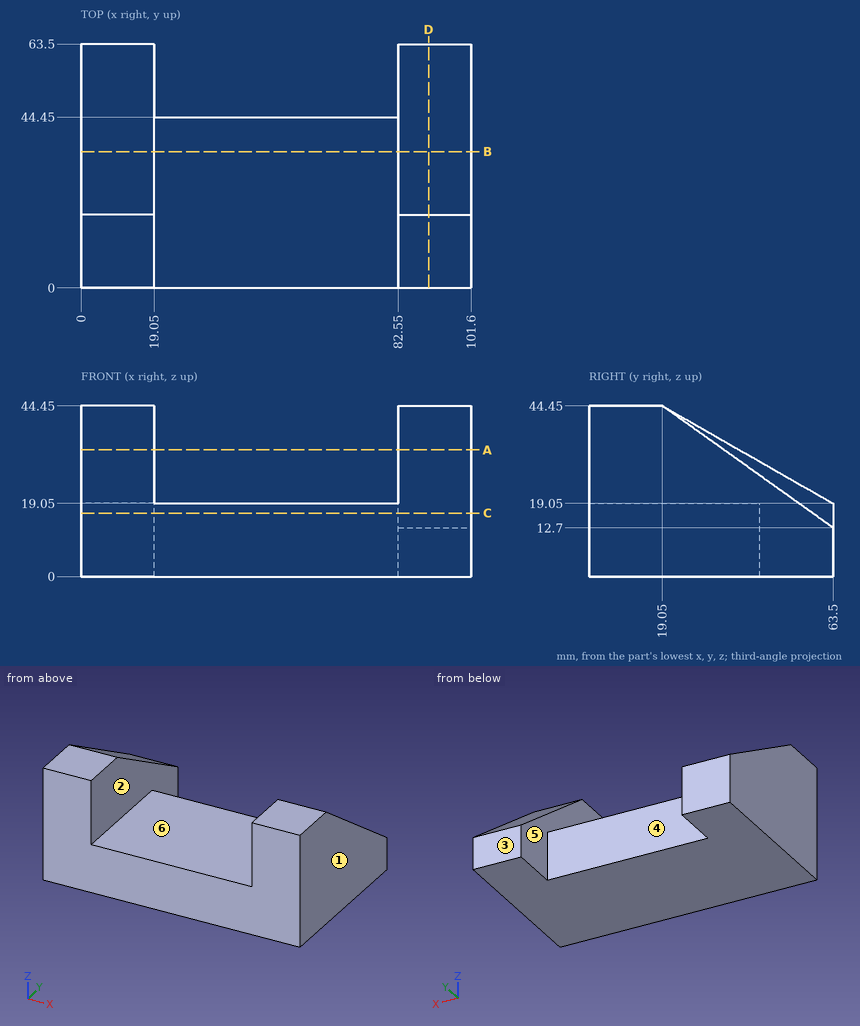
Design review of the part shown in the three views and the two pictorial views. Dimensions are in mm from the part's minimum x, y and z. A direction names the side the tool comes from. Give positions to 0.01 mm unless a question says otherwise; leave off trailing zeros. Loops run counter-clockwise (first coordinate to the right, second up) from the corner with the lowest first, then second, coordinate; pieces in that order, holes last. Notation, with made-up numbers: M 21.5,-18.5 L 71.5,-18.5 A20 cw 71.5,10.5 Z; hole C -36,-23 d3. An arc over 180 degrees is marked long. Answer as a JSON object with one key per item and string values. Group by question number.
Q1. For probe 1 along X at (y, z) = (16, 20.5); probe 2 along Y at (x, z) = (35.5, 10); probe 3 along Z at (x, y) = (81.5, 34), list the stretches that pass through material, from the lowest coordinate up. Write a range as [from, to].
Q2. Add section C-C on z = 16.5. Give the boundary of the cut face in (x, y), and give its area (3 significant figures).
Q3. Mouldability with a two-part tool opening along X and no side actions: class the marked faces 1, 2 and 3 as +X half, -X half, draft (parallel to the pull), parting line (faces both ways), or undercut.
Q4. Add section B-B on y = 35.5. Give the boundary of the cut face in (x, z).
Q5. Add section A-A on z = 33. Give the boundary of the cut face in (x, y), and give its area (3 significant figures).
Q6. Insertion check: P1, Ø5.5, axis at x = 43.5, z = 11, coming from the +Y side. The pin has a flat end and moves straight along its axis. Give the tip position at first contact, or say it passes through.
Q7. Add section D-D on x = 90.5. Give the boundary of the cut face in (y, z).
Q8. Tool access review of the marked faces 4, 5 and 6: name each direction out of +Z, -Z, +X, -X, +Y, -Y from which nothing blocks a thin tool from reaching the whole face with its end or side.
Checked values:
{
 "1": {"probe 1": "[0, 19.05], [82.55, 101.6]", "probe 2": "[0, 44.45]", "probe 3": "[0, 19.05]"},
 "2": {"outline": "M 0,0 L 101.6,0 L 101.6,58.18 L 82.55,58.18 L 82.55,44.45 L 19.05,44.45 L 19.05,63.5 L 0,63.5 Z", "area": "5,140 mm²"},
 "3": {"face 1": "+X half", "face 2": "undercut", "face 3": "draft"},
 "4": {"outline": "M 0,0 L 101.6,0 L 101.6,32.7 L 82.55,32.7 L 82.55,19.05 L 19.05,19.05 L 19.05,35.05 L 0,35.05 Z"},
 "5": {"outline": "M 0,0 L 19.05,0 L 19.05,39.09 L 0,39.09 Z; M 82.55,0 L 101.6,0 L 101.6,35.08 L 82.55,35.08 Z", "area": "1,410 mm²"},
 "6": {"P1": "y = 44.45"},
 "7": {"outline": "M 0,0 L 63.5,0 L 63.5,12.7 L 19.05,44.45 L 0,44.45 Z"},
 "8": {"face 4": "+Z, -Z, +Y", "face 5": "+Z, +Y", "face 6": "+Z, +Y, -Y"}
}
